```python
from build123d import *

# Parameters (mm, degrees)
ESBO_O1_W                = 174
ESBO_O1_H                = 75.81
RESSALTO_EXTRUS_O1_DEPTH = 3
ESBO_O3_W                = 3
ESBO_O3_H                = 12.635
RESSALTO_EXTRUS_O2_DEPTH = 3
ESBO_O4_W                = 3
ESBO_O4_H                = 12.635
RESSALTO_EXTRUS_O3_DEPTH = 3


with BuildPart() as part:
    # Esboço1 → Ressalto-extrusão1 (new body)
    with BuildSketch(Plane.XY):
        Rectangle(ESBO_O1_W, ESBO_O1_H)
    extrude(amount=RESSALTO_EXTRUS_O1_DEPTH)

    # Esboço3 → Ressalto-extrusão2 (add)
    with BuildSketch(Plane.XY.offset(3)):
        with Locations((-88.5, 6.3175)):
            Rectangle(ESBO_O3_W, ESBO_O3_H)
        with Locations((-88.5, 31.5875)):
            Rectangle(ESBO_O3_W, ESBO_O3_H)
        with Locations((-88.5, -18.9525)):
            Rectangle(ESBO_O3_W, ESBO_O3_H)
    extrude(amount=-RESSALTO_EXTRUS_O2_DEPTH)

    # Esboço4 → Ressalto-extrusão3 (add)
    with BuildSketch(Plane.XY.offset(3)):
        with Locations((88.5, 18.9525)):
            Rectangle(ESBO_O4_W, ESBO_O4_H)
        with Locations((88.5, -6.3175)):
            Rectangle(ESBO_O4_W, ESBO_O4_H)
        with Locations((88.5, -31.5875)):
            Rectangle(ESBO_O4_W, ESBO_O4_H)
    extrude(amount=-RESSALTO_EXTRUS_O3_DEPTH)


solid = part.part
```
Model file for the job. Use its own axes, mm. A direction names the side the tool comes from. Coordinates: 2 decimals unless noted, no trailing zeros. Order: outer loops, then holes, each group sorted by start corner. A loop starts at its lowest first (then second) coordinate and runs counter-clockwise, first axis right, second up. Notation, with made-up numbers: (-14, 52.25) - (36, 52.25) arc R36 cw to (36, 86.25) - close; hole circle Ø10 at (-5, 17.5). An arc over 180 degrees is marked (long way). Return JSON: item names as keys, results as strings. Group by question number.
1) Saw through at B-B, the plane y = 2. Write the cut outline in (x, z).
2) Probe line 1 (X direction, y = 4, z = 1.8); line 2 (X direction, y = -29, z = 2.5). List the from-to ranges inside material, lowest first. Write a range as from..to.
3) Tool access for faces 1 (the flat face through (-1, 1, 0)), 2 (the flat face through (87, -19, 1)), 3 (the flat face through (-89, 25.27, 2)): list every direction of +Z, -Z, +X, -X, +Y, -Y with a clear straight run to the whole face (end or side of a thin tool).
4) Mould opens along Y. For faces 4 (the flat face through (-87, -32, 1)), 5 (the flat face through (88, 25.27, 2)), 6 (the flat face through (-87, 19, 1)) say: released by +Y, released by -Y, zero draft, split by the parting line, or undercut.
5) Flat gauge pins, fed straight in: P1, Ø0.9, axis at x = -88, z = 2, coming from the -Y side; P2, Ø0.9, axis at x = 88, z = 2, coming from the +Y side; P3, Ø0.9, axis at y = -20.5, z = 1.5, coming from the +X side. Where does each tip first touch, or does it go through?
6) Saw through at A-A, the plane z = 1.8. Write the cut outline in (x, y) (3 decimals).
Values found:
{
 "1": {"outline": "(-90, 0) - (87, 0) - (87, 3) - (-90, 3) - close"},
 "2": {"line 1": "x = -90..87", "line 2": "x = -87..90"},
 "3": {"face 1": "-Z, +X, -X, +Y, -Y", "face 2": "+Z, -Z, +X", "face 3": "+Z, -Z, -X"},
 "4": {"face 4": "zero draft", "face 5": "released by +Y", "face 6": "undercut"},
 "5": {"P1": "stops at y = -25.27", "P2": "stops at y = 25.27", "P3": "stops at x = 87"},
 "6": {"outline": "(-90, -25.27) - (-87, -25.27) - (-87, -37.905) - (90, -37.905) - (90, -25.27) - (87, -25.27) - (87, -12.635) - (90, -12.635) - (90, 0) - (87, 0) - (87, 12.635) - (90, 12.635) - (90, 25.27) - (87, 25.27) - (87, 37.905) - (-90, 37.905) - (-90, 25.27) - (-87, 25.27) - (-87, 12.635) - (-90, 12.635) - (-90, 0) - (-87, 0) - (-87, -12.635) - (-90, -12.635) - close"}
}
